Could you check a few things on this model? Use its own coordinates, in mm. Give positions to 0.01 mm unless a question says otherwise; leave off trailing zeros. Order: outer loops, then holes, each group sorted by start corner. A loop starts at its lowest first (then second) coordinate and runs counter-clockwise, first axis right, second up.
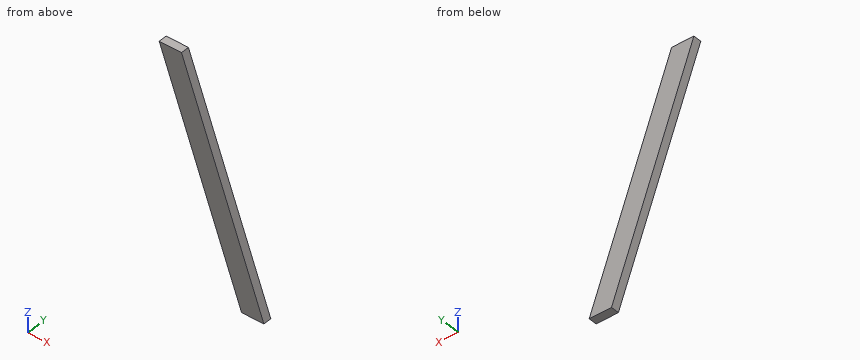
from build123d import *

# Parameters (mm, degrees)
BOX016_W               = 60
BOX016_H               = 24
BOX016_DEPTH           = 827
BOX016_PITCH_ANGLE     = 19.999975
BOX016_PLACEMENT_ANGLE = 180
BOX015_W               = 300
BOX015_H               = 24
BOX015_DEPTH           = 648


with BuildPart() as cube007:
    # Box016 → Box016 (new body)
    with BuildSketch(Plane.XY):
        with Locations((30, 12)):
            Rectangle(BOX016_W, BOX016_H)
    extrude(amount=BOX016_DEPTH)


with BuildPart() as cube007_1:
    # Box016 pitch: moved
    add(cube007.part.rotate(Axis((0, 0, 0), (0, 1, 0)), BOX016_PITCH_ANGLE))


with BuildPart() as cube007_2:
    # Box016 placement: moved
    add(cube007_1.part.moved(Location((300, 24, 24))).rotate(Axis((300, 24, 24), (0, 0, 1)), BOX016_PLACEMENT_ANGLE))


with BuildPart() as stand:
    # Box015 → Box015 (new body)
    with BuildSketch(Plane.XY.offset(24)):
        with Locations((150, 12)):
            Rectangle(BOX015_W, BOX015_H)
    extrude(amount=BOX015_DEPTH)

    # Common: intersect Cube007
    add(cube007_2.part, mode=Mode.INTERSECT)


solid = stand.part
Item 1: Imagine slicing it at A-A on y = 12.5. List the corners of the cut face in (x, z) for me.
Findings:
outline: (0.3, 672) - (236.15, 24) - (300, 24) - (64.15, 672) - close
Item 2: For pin 1 (2 mm diameter, centred on y = 10, z = 440, fed in from -X); pin 2 (12 mm diameter, centred on y = 13.5, z = 333, fed in from +X); pin 3 (6 mm diameter, centred on y = 18.5, z = 469, fed in from -X), each with a flat end and sliding along its axis, tell me the tip position at first contact or that it passes through.
Findings:
pin 1: stops at x = 84.37
pin 2: stops at x = 189.72
pin 3: stops at x = 73.09
Item 3: Imagine slicing it at B-B on x = 199. List the corners of the cut face in (y, z) for me.
Findings:
outline: (0, 126.07) - (24, 126.07) - (24, 301.5) - (0, 301.5) - close
Item 4: Please list where these lines run through material, in increasing order: line 1 along X through (y, z) = (23, 461.5); line 2 along X through (y, z) = (2.25, 315.5).
Findings:
line 1: x = 76.91 to 140.76
line 2: x = 130.05 to 193.9
